Autodesk Inventor part; units mm, degrees
ref_plane "YZ Plane" through (0, 0, 0) normal (1, 0, 0) x (0, 1, 0)
ref_plane "XZ Plane" through (0, 0, 0) normal (0, 1, 0) x (-1, 0, 0)
ref_plane "XY Plane" through (0, 0, 0) normal (0, 0, 1) x (1, 0, 0)
sketch "スケッチ1" plane through (0, 0, 0) normal (1, 0, 0) x (0, 1, 0)
  line L0 (0, 0) -> (3, 0)
  line L1 (3, 0) -> (3, 3)
  line L2 (3, 3) -> (0, 3)
  line L3 (0, 3) -> (0, 0)
  line L4 (0, 0) -> (4, 0)
  line L5 (4, 0) -> (4, -37)
  line L6 (4, -37) -> (0, -37)
  line L7 (0, -37) -> (0, 0)
  line L8 (0, -37) -> (3, -37)
  line L9 (3, -37) -> (3, -40)
  line L10 (3, -40) -> (0, -40)
  line L11 (0, -40) -> (0, -37)
  dimension "d0" = 3
  dimension "d1" = 3
  dimension "d2" = 4
  dimension "d3" = 37
  dimension "d4" = 3
  dimension "d5" = 3
revolve "回転1" add sketch "スケッチ1" angle 360 about axis through (0, 0, -37) along (0, 0, 1)
sketch "スケッチ2" plane through (0, 0, 0) normal (0, 0, 1) x (1, 0, 0)
  circle A0 centre (0, 0) radius 4
  point P0 (0, 4)
ref_plane "作業平面1" through (0, 4, 0) normal (0, 1, 0) x (-1, 0, 0)
sketch "スケッチ3" plane through (0, 4, 0) normal (0, 1, 0) x (-1, 0, 0)
  line L0 (0, 0) -> (0, 3)
  line L1 (3, 3) -> (-3, 3)
  line L2 (1.5, -3) -> (-1.5, -3)
  line L3 (-1.5, -3) -> (-1.5, -8)
  line L4 (-1.5, -8) -> (1.5, -8)
  line L5 (1.5, -8) -> (1.5, -3)
  line L6 (4, 0) -> (-4, 0)
  circle A0 centre (0, -3) radius 1.5
  circle A1 centre (0, -8) radius 1.5
  line L7 (-1.5, -27) -> (1.5, -27)
  line L8 (1.5, -27) -> (1.5, -17)
  line L9 (1.5, -17) -> (-1.5, -17)
  line L10 (-1.5, -17) -> (-1.5, -27)
  circle A2 centre (0, -27) radius 1.5
  circle A3 centre (0, -17) radius 1.5
  dimension "d7" = 3
  dimension "d8" = 5
  dimension "d9" = 3
  dimension "d12" = 3
  dimension "d13" = 9
  dimension "d14" = 10
extrude "押し出し1" cut sketch "スケッチ3" against normal blind 1.8
properties part number "入力軸" material "鋼、炭素鋼"
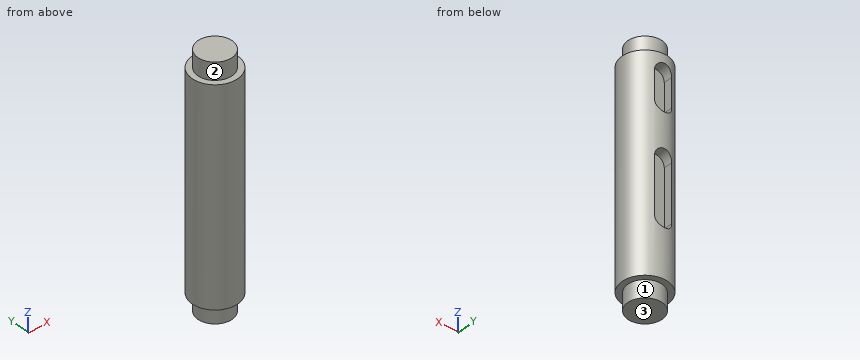
Source: CAD feature listing. Evaluate the final solid. Frame: model axes, mm. Face numbers are marked on the shaded views. A direction names the side the tool comes from. Give positions to 0.01 mm unless a question says otherwise; leave off trailing zeros. Write each loop counter-clockwise with the first axis right and the second up, starting at its lowest first coordinate (ties: lowest second). Pieces come first, ordered by that corner, then holes. Notation, with made-up numbers: (53, -35) - (72, -35) arc R34 ccw to (72, -2) - close; hole circle Ø5 at (4, 14). An arc over 180 degrees is marked (long way). Write item = value, one per line. Start each with the question number.
Q1. Cut plane A-A, the plane x = 0. Return loops of the section in (y, z), then the cut area to 3 significant figures.
Q2. Pin query (flat end, axial travel): pin 1 Ø1.5 at (x, z) = (0.5, -22.5) entering from +Y; pin 2 Ø2 at (x, z) = (1.5, -14.5) entering from -Y; pin 3 Ø1.7 at (y, z) = (3, -4.5) entering from +X. Return the tip coordinate at first contact, or that it passes through.
Q3. Cut plane C-C, the plane z = -25. Return loops of the section in (x, y).
Q4. Cut plane B-B, the plane y = 0. Return loops of the section in (x, z), then the cut area to 3 significant figures.
Q5. Cut plane D-D, the plane x = -2.25. Return loops of the section in (y, z).
Q6. Material intervals for probe 1 along Z at (x, y) = (2.25, -2.75); probe 2 along Y at (x, z) = (-0.25, -30); probe 3 along X at (y, z) = (-0.5, -30), sorted ascending.
Q7. Reachability of the marked faces 1, 2 and 3 from +Z, -Z, +X, -X, +Y, -Y: full face, straight path, thin tool, end or side. Return the list, or none.
Computed values:
q1.outline = (-4, -37) - (-3, -37) - (-3, -40) - (3, -40) - (3, -37) - (4, -37) - (4, -28.5) - (2.2, -28.5) - (2.2, -15.5) - (4, -15.5) - (4, -9.5) - (2.2, -9.5) - (2.2, -1.5) - (4, -1.5) - (4, 0) - (3, 0) - (3, 3) - (-3, 3) - (-3, 0) - (-4, 0) - close
q1.area = 294 mm²
q2.pin_1 = 2.2
q2.pin_2 = -3.97
q2.pin_3 = 3.37
q3.outline = (-1.5, 2.2) - (-1.5, 3.71) arc R4 ccw (long way) to (1.5, 3.71) - (1.5, 2.2) - close
q4.outline = (-4, -37) - (-3, -37) - (-3, -40) - (3, -40) - (3, -37) - (4, -37) - (4, 0) - (3, 0) - (3, 3) - (-3, 3) - (-3, 0) - (-4, 0) - close
q4.area = 332 mm²
q5.outline = (-3.31, -37) - (-1.98, -37) - (-1.98, -40) - (1.98, -40) - (1.98, -37) - (3.31, -37) - (3.31, 0) - (1.98, 0) - (1.98, 3) - (-1.98, 3) - (-1.98, 0) - (-3.31, 0) - close
q6.probe_1 = -37 to 0
q6.probe_2 = -3.99 to 3.99
q6.probe_3 = -3.97 to 3.97
q7.face_1 = -Z
q7.face_2 = +Z
q7.face_3 = -Z, +X, -X, +Y, -Y
